Work out the finished part from the listing and answer in its coordinate system (mm). A direction names the side the tool comes from. Coordinates: 2 decimals unless noted, no trailing zeros. Loops run counter-clockwise (first coordinate to the right, second up) from the corner with the lowest first, then second, coordinate; pieces in that order, holes last.
Autodesk Fusion 360 part; units mm, degrees
box "BoxPrimitive1" add length 25 width 16 height 18 placed x (0, 1, 0) y (0, 0, 1) z (1, 0, 0) at (0, 0, 0)
sketch "Sketch2" plane through (18, 0, 0) normal (1, 0, 0) x (0, 0, -1)
  line L0 (0, 25) -> (-16, 25)
  line L1 (-16, 25) -> (-16, 0)
  line L2 (-16, 0) -> (0, 0)
  line L3 (0, 0) -> (0, 25)
  line L4 (-8, 25) -> (-8, 13.5) construction
  line L5 (-1.85, 25) -> (-14.15, 25)
  line L6 (-14.15, 25) -> (-14.15, 2)
  line L7 (-14.15, 2) -> (-1.85, 2)
  line L8 (-1.85, 2) -> (-1.85, 25)
  line L9 (-1.85, 25) -> (-14.15, 2) construction
  line L10 (-14.15, 25) -> (-1.85, 2) construction
  point P0 (-8, 13.5)
  dimension "d12" = 11.5
  dimension "d13" = 12.3
  dimension "d14" = 23
extrude "Extrude1" cut sketch "Sketch2" against normal blind 16.5 contours L0 L5 L6 L7 L8
equation "Height = 25 mm"
equation "Width = 16 mm"
equation "LengthHole = 16.5 mm"
equation "Length = 18 mm"
equation "d5 = Height"
equation "d6 = Width"
equation "d7 = Length"
equation "WidthHole = 12.3 mm"
equation "Heighthole = 23 mm"
equation "d12 = Heighthole / 2"
equation "d13 = WidthHole"
equation "d14 = Heighthole"
1. A cutting plane is placed at A-A, the plane x = 11.5. Give the vertices of the cut face in (y, z), then the cut area to 3 significant figures.
2. Each of these flat-tipped pins is pushed along its axis until it touches: P1, Ø10, axis at x = 11.5, y = 17, coming from the -Z side; P2, Ø4, axis at y = 17.5, z = 8.5, coming from the +X side. Where does it stop, or does it pass through?
3. For faces 1 (the flat face through (1, 25, 7)), 2 (the flat face through (1.5, 14, 8)), determine the directions among +Z, -Z, +X, -X, +Y, -Y from which every point of the face is accessible in a straight line to the end or side of a thin tool.
4. Straight lines are drawn through the part: probe 1 along Z at (x, y) = (16.25, 15.25); probe 2 along Y at (x, z) = (8.25, 2.5); probe 3 along X at (y, z) = (16, 5). For each, find the intervals that lie inside material, in ascending order.
5. A cutting plane is placed at C-C, the plane z = 7. Give the vertices of the cut face in (x, y), then the cut area to 3 significant figures.
6. A cutting plane is placed at B-B, the plane y = 19. Give the vertices of the cut face in (x, z), then the cut area to 4 significant figures.
Answers below:
1. outline: (0, 0) - (25, 0) - (25, 1.85) - (2, 1.85) - (2, 14.15) - (25, 14.15) - (25, 16) - (0, 16) - close
1. area: 117 mm2
2. P1: stops at z = 0
2. P2: stops at x = 1.5
3. face 1: +Z, -Z, +X, -X, +Y
3. face 2: +X, +Y
4. probe 1: z = 0 to 1.85, 14.15 to 16
4. probe 2: y = 0 to 2
4. probe 3: x = 0 to 1.5
5. outline: (0, 0) - (18, 0) - (18, 2) - (1.5, 2) - (1.5, 25) - (0, 25) - close
5. area: 70.5 mm2
6. outline: (0, 0) - (18, 0) - (18, 1.85) - (1.5, 1.85) - (1.5, 14.15) - (18, 14.15) - (18, 16) - (0, 16) - close
6. area: 85.05 mm2
